Source: CAD feature listing. Evaluate the final solid. Frame: model axes, mm. Round coordinates to 2 decimals unless told otherwise and drop trailing zeros. Loops run counter-clockwise (first coordinate to the right, second up) from the corner with the lowest first, then second, coordinate; pieces in that order, holes last.
(1) Section B-B, the plane z = -120. Return the cut outline in (x, y), plus the area to 3 significant figures.
(2) Section C-C, the plane y = 2.5. Count the separate pieces of the cut face and the enclosed holes in it, plus the area to 3 significant figures.
(3) Section D-D, the plane z = -77.5. Return the cut outline in (x, y).
(4) Section A-A, the plane x = 10. Return the cut outline in (y, z), plus the area to 3 significant figures.
(5) Material intervals for probe 1 along X at (y, z) = (4, -52.5); probe 2 along Z at (x, y) = (77.5, 7.2); probe 3 along Z at (x, y) = (53, 5.5), sorted ascending.
(6) First-contact query: pin 1 Ø6.5 at (x, z) = (10, -120) entering from -Y; pin 2 Ø8.5 at (x, z) = (53.5, -52) entering from -Y. Flat tips, straight axial feed; report the tip coordinate or a pass-through.
```python
from build123d import *

# Parameters (mm, degrees)
SKETCH_1_W          = 130
SKETCH_1_H          = 130
EXTRUDE_1_DEPTH     = 7.5
HOLE_WIZARD_M6_2_D  = 5
SKETCH_6_R          = 5.4
CUT_EXTRUDE_1_DEPTH = 6.5
SKETCH_7_R          = 3.3
CUT_EXTRUDE_2_DEPTH = 2


with BuildPart() as part:
    # 草图1 → 凸台-拉伸1 (new body)
    with BuildSketch(Plane(origin=(0, 0, 0), x_dir=(1, 0, 0), z_dir=(0, 1, 0))):
        with Locations((65, 65)):
            Rectangle(SKETCH_1_W, SKETCH_1_H)
    extrude(amount=EXTRUDE_1_DEPTH)

    # M6 螺纹孔2 (through all)
    with Locations(Plane(origin=(10, 7.5, -120), x_dir=(0, 0, 1), z_dir=(0, 1, 0))):
        with Locations((0, 0), (0, 110), (110, 110), (110, 0)):
            Hole(HOLE_WIZARD_M6_2_D / 2)

    # 草图6 → 切除-拉伸1 (cut)
    with BuildSketch(Plane(origin=(0, 0, 0), x_dir=(-1, 0, 0), z_dir=(0, -1, 0))):
        with Locations((-52.5, 52.5)):
            Circle(SKETCH_6_R)
        with Locations((-77.5, 52.5)):
            Circle(SKETCH_6_R)
        with Locations((-52.5, 77.5)):
            Circle(SKETCH_6_R)
        with Locations((-77.5, 77.5)):
            Circle(SKETCH_6_R)
    extrude(amount=-CUT_EXTRUDE_1_DEPTH, mode=Mode.SUBTRACT)

    # 草图7 → 切除-拉伸2 (cut, through all)
    with BuildSketch(Plane.XZ.offset(-6.5)):
        with Locations((52.5, -52.5)):
            Circle(SKETCH_7_R)
        with Locations((77.5, -52.5)):
            Circle(SKETCH_7_R)
        with Locations((77.5, -77.5)):
            Circle(SKETCH_7_R)
        with Locations((52.5, -77.5)):
            Circle(SKETCH_7_R)
    extrude(amount=-CUT_EXTRUDE_2_DEPTH, mode=Mode.SUBTRACT)


solid = part.part
```
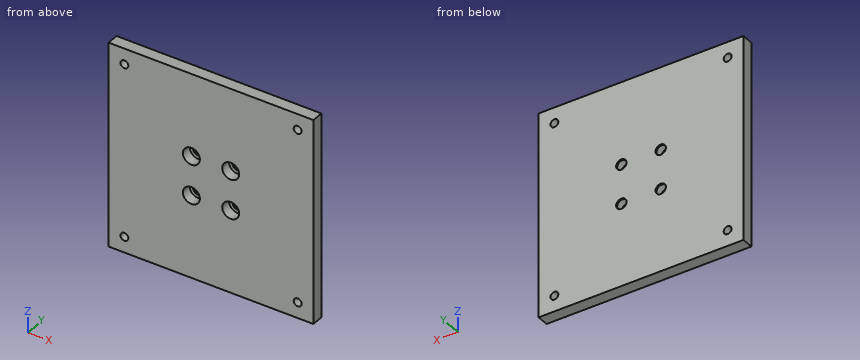
Output values:
1. outline: (0, 0) - (7.5, 0) - (7.5, 7.5) - (0, 7.5) - close; (12.5, 0) - (117.5, 0) - (117.5, 7.5) - (12.5, 7.5) - close; (122.5, 0) - (130, 0) - (130, 7.5) - (122.5, 7.5) - close
1. area: 900 mm2
2. separate pieces: 1
2. enclosed holes: 8
2. area: 16,500 mm2
3. outline: (0, 0) - (47.1, 0) - (47.1, 6.5) - (49.2, 6.5) - (49.2, 7.5) - (0, 7.5) - close; (55.8, 6.5) - (57.9, 6.5) - (57.9, 0) - (72.1, 0) - (72.1, 6.5) - (74.2, 6.5) - (74.2, 7.5) - (55.8, 7.5) - close; (80.8, 6.5) - (82.9, 6.5) - (82.9, 0) - (130, 0) - (130, 7.5) - (80.8, 7.5) - close
4. outline: (0, -130) - (7.5, -130) - (7.5, -122.5) - (0, -122.5) - close; (0, -117.5) - (7.5, -117.5) - (7.5, -12.5) - (0, -12.5) - close; (0, -7.5) - (7.5, -7.5) - (7.5, 0) - (0, 0) - close
4. area: 900 mm2
5. probe 1: x = 0 to 47.1, 57.9 to 72.1, 82.9 to 130
5. probe 2: z = -130 to -80.8, -74.2 to -55.8, -49.2 to 0
5. probe 3: z = -130 to -82.88, -72.12 to -57.88, -47.12 to 0
6. pin 1: stops at y = 0
6. pin 2: stops at y = 6.5
